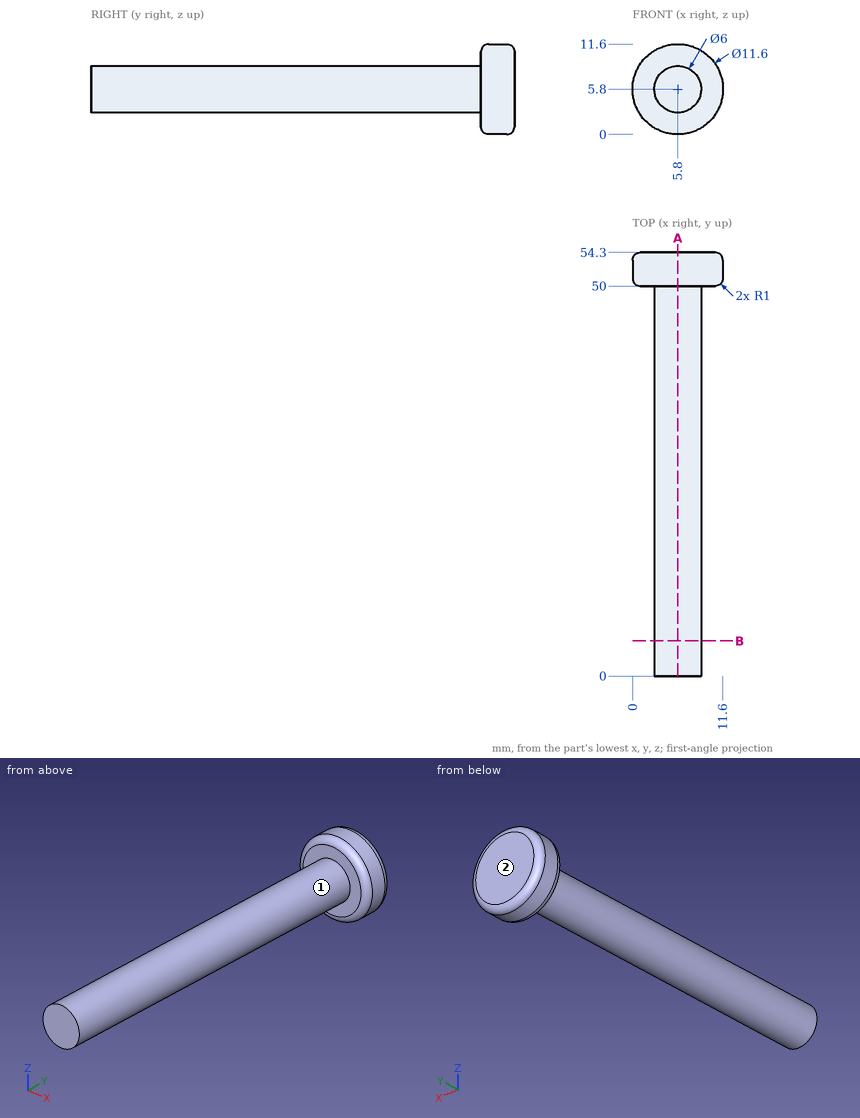
The figure shows three views and two pictorial views of one solid part (mm, origin at its lowest corner). Answer the questions. A direction names the side the tool comes from. Coordinates: 2 decimals unless noted, no trailing zeros. Loops run counter-clockwise (first coordinate to the right, second up) from the corner with the lowest first, then second, coordinate; pieces in that order, holes last. Notation, with made-up numbers: (-4, 73.25) -> (26, 73.25) arc R17 cw to (26, 81.25) -> close; hole circle Ø2 at (87.25, -18). An arc over 180 degrees is marked (long way). Return JSON: item names as keys, results as strings. Group by question number.
(1) Which of the six approach directions +Z, -Z, +X, -X, +Y, -Y give full straight-line access (tool end or side, diameter ignored) to the marked faces 1 and 2?
(2) A cutting plane is placed at A-A on x = 5.8. Write down the section's boundary in (y, z).
(3) Given pin 1 Ø6 at (x, z) = (10, 10.5) entering from -Y; pin 2 Ø2 at (y, z) = (7, 5.5) entering from +X; pin 3 Ø4 at (x, y) = (3.5, 27) entering from -Z; pin 4 Ø2 at (y, z) = (48.5, 10) entering from -X, each flat-ended and moving along its own axis, determine where each tip first touches the part or whether it passes through.
(4) A cutting plane is placed at B-B on y = 4.5. Write down the section's boundary in (x, z), and give its area (3 significant figures).
(5) Find the intervals of material crossed by probe 1 along Z at (x, y) = (5.75, 30); probe 2 along Y at (x, z) = (9.5, 8.5), in increasing order. Write a range as from..to.
The answers:
{
 "1": {"face 1": "-Y", "face 2": "+Z, -Z, +X, -X, +Y"},
 "2": {"outline": "(0, 2.8) -> (50, 2.8) -> (50, 1) arc R1 ccw to (51, 0) -> (53.3, 0) arc R1 ccw to (54.3, 1) -> (54.3, 10.6) arc R1 ccw to (53.3, 11.6) -> (51, 11.6) arc R1 ccw to (50, 10.6) -> (50, 8.8) -> (0, 8.8) -> close"},
 "3": {"pin 1": "stops at y = 50", "pin 2": "stops at x = 8.8", "pin 3": "stops at z = 2.82", "pin 4": "passes through"},
 "4": {"outline": "circle Ø6 at (5.8, 5.8)", "area": "28.3 mm^2"},
 "5": {"probe 1": "z = 2.8..8.8", "probe 2": "y = 50..54.3"}
}
